Verification items for the finished model (mm, model axes). A direction names the side the tool comes from. Give positions to 0.01 mm unless a question says otherwise; leave off trailing zeros. Loops run counter-clockwise (first coordinate to the right, second up) from the corner with the lowest first, then second, coordinate; pieces in that order, holes last. Notation, with made-up numbers: M 35.25,35 L 87.25,35 A27 ccw 87.25,74 Z; hole C 22,17 d10. An arc over 180 degrees is marked long. Answer in a Markdown table with one row per item.
```python
from build123d import *

# Parameters (mm, degrees)
EXTRUDE_1_DEPTH     = 36
SKETCH_2_R          = 1.5
CUT_EXTRUDE_1_DEPTH = 39.678159212


with BuildPart() as part:
    # 草图1 → 凸台-拉伸1 (new body)
    with BuildSketch(Plane.XY):
        with BuildLine():
            Line((-1.414213562, 0.5), (-14, 0.5))
            Line((-14, 0.5), (-14, -0.5))
            Line((-14, -0.5), (-1.414213562, -0.5))
            ThreePointArc((-1.414213562, -0.5), (1.5, 0), (-1.414213562, 0.5))
        make_face()
    extrude(amount=EXTRUDE_1_DEPTH)

    # 草图2 → 切除-拉伸1 (cut, through all)
    with BuildSketch(Plane(origin=(0, 0.5, 0), x_dir=(1, 0, 0), z_dir=(0, 1, 0))):
        with Locations(Location((-7.914213562, -5.5, 0), (0, 0, 180))):
            Circle(SKETCH_2_R)
        with Locations(Location((-7.914213562, -30.5, 0), (0, 0, 270))):
            Circle(SKETCH_2_R)
    extrude(amount=-CUT_EXTRUDE_1_DEPTH, mode=Mode.SUBTRACT)


solid = part.part
```
Item 1: Release check for a two-part mould opening along Z. For faces 1 (the cylindrical face through (-9.345, 0.007, 5.951)), 2 (the flat face through (-14, 0, 18)), 3 (the flat face through (-5, 0, 36)) record: released by +Z, released by -Z, zero draft, split by the parting line, or undercut.
Reported:
| item | result |
|---|---|
| face 1 | undercut |
| face 2 | zero draft |
| face 3 | released by +Z |
Item 2: Sectioned sample at D-D (z = 25). Record the cut outline in (x, y), and give its area (3 significant figures).
Reported:
| item | result |
|---|---|
| outline | M -14,-0.5 L -1.41,-0.5 A1.5 ccw long -1.41,0.5 L -14,0.5 Z |
| area | 19.6 mm^2 |
Item 3: Sectioned sample at B-B (x = -7). Record the cut outline in (y, z).
Reported:
| item | result |
|---|---|
| outline | M -0.5,0 L 0.5,0 L 0.5,4.31 L -0.5,4.31 Z; M -0.5,6.69 L 0.5,6.69 L 0.5,29.31 L -0.5,29.31 Z; M -0.5,31.69 L 0.5,31.69 L 0.5,36 L -0.5,36 Z |
Item 4: Tool access check on faces 4 (the cylindrical face through (1.5, -0.06, 17.75)), 5 (the flat face through (-8, -0.5, 18)), 6 (the flat face through (-8, 0.5, 18)). Record the directions out of +Z, -Z, +X, -X, +Y, -Y that give a thin tool (end or side, any length) a straight path to the whole face; none if there is none.
Reported:
| item | result |
|---|---|
| face 4 | +Z, -Z |
| face 5 | +Z, -Z, -X, -Y |
| face 6 | +Z, -Z, -X, +Y |
Item 5: Sectioned sample at C-C (y = 0). Record the cut outline in (x, z).
Reported:
| item | result |
|---|---|
| outline | M -14,0 L 1.5,0 L 1.5,36 L -14,36 Z; hole C -7.91,5.5 d3; hole C -7.91,30.5 d3 |
Item 6: Scan lines: L1, parallel to X at y = 0, z = 30.5; L2, parallel to Y at x = -10, z = 11; L3, parallel to X at y = 0.1, z = 18. Record each from-to range of solid material in increasing order. Write a range as [from, to].
Reported:
| item | result |
|---|---|
| L1 | x = [-14, -9.41], [-6.41, 1.5] |
| L2 | y = [-0.5, 0.5] |
| L3 | x = [-14, 1.5] |
Item 7: Go/stop test with flat-tipped pins: pin 1 (4 mm diameter, centred on x = -7.91, z = 30.5, fed in from +Y); pin 2 (4 mm diameter, centred on x = -7.91, z = 5.5, fed in from -Y). Record where each tip stops, or that it passes through.
Reported:
| item | result |
|---|---|
| pin 1 | stops at y = 0.5 |
| pin 2 | stops at y = -0.5 |
Item 8: Sectioned sample at A-A (z = 5.5). Record the cut outline in (x, y), and give its area (3 significant figures).
Reported:
| item | result |
|---|---|
| outline | M -14,-0.5 L -9.41,-0.5 L -9.41,0.5 L -14,0.5 Z; M -6.41,-0.5 L -1.41,-0.5 A1.5 ccw long -1.41,0.5 L -6.41,0.5 Z |
| area | 16.6 mm^2 |
